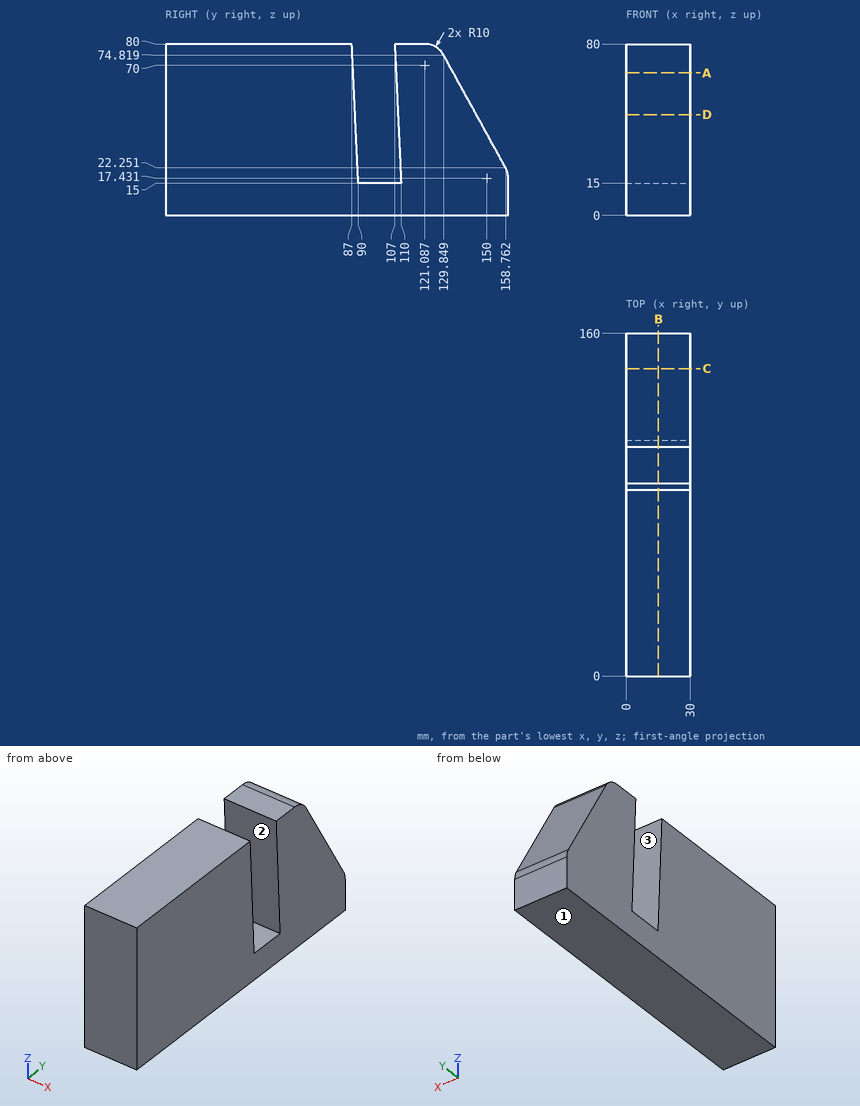
For this review, use the dimensioned drawing (mm, ordinates from the lowest corner) and the shaded views. Give positions to 0.01 mm unless a question says otherwise; leave off trailing zeros. Order: outer loops, then holes, each group sorted by start corner. A loop starts at its lowest first (then second) coordinate and runs counter-clockwise, first axis right, second up. Notation, with made-up numbers: M -29,30 L 28,30 A17 cw 28,35 Z; hole C -32.75,-23 d6. An arc over 180 degrees is marked long. One line per question, with ' | ' between items. Start each with the question number.
1) Mouldability with a two-part tool opening along Z and no side actions: class the marked faces 1, 2 and 3 as pulls with the +Z half, pulls with the -Z half, needs draft (parallel to the pull), parting line crosses it, or undercut.
2) Consider section D-D, the plane z = 47. Give the boundary of the cut face in (x, y), then the cut area to 3 significant figures.
3) Consider section B-B, the plane x = 15. Give the boundary of the cut face in (y, z), then the cut area to 3 significant figures.
4) Clearance check with flat-ended pins moving along their axes: P1, Ø10, axis at x = 10, z = 32.5, coming from the +Y side (1 decimal); P2, Ø5, axis at x = 25, z = 63.5, coming from the +Y side. State where each tip first meets the part, or that it passes through.
5) Consider section A-A, the plane z = 66.5. Give the boundary of the cut face in (x, y) (1 decimal).
6) Wall thickness on L1, parallel to Y at x = 11.25, z = 69; L2, parallel to Y at x = 9.25, z = 46; L3, parallel to Z at x = 18, y = 106.5: over which ranges is each line inside the solid? List them lowest first. Write a range as from..to.
7) Consider section C-C, the plane y = 143.5. Give the boundary of the cut face in (x, z), then the cut area to 3 significant figures.
Found:
1) face 1: pulls with the -Z half | face 2: undercut | face 3: pulls with the +Z half
2) outline: M 0,0 L 30,0 L 30,88.52 L 0,88.52 Z; M 0,108.52 L 30,108.52 L 30,145.15 L 0,145.15 Z | area: 3,750 mm²
3) outline: M 0,0 L 160,0 L 160,17.43 A10 ccw 158.76,22.25 L 129.85,74.82 A10 ccw 121.09,80 L 107,80 L 110,15 L 90,15 L 87,80 L 0,80 Z | area: 10,500 mm²
4) P1: stops at y = 155.9 | P2: stops at y = 137.45
5) outline: M 0,0 L 30,0 L 30,87.6 L 0,87.6 Z; M 0,107.6 L 30,107.6 L 30,134.4 L 0,134.4 Z
6) L1: y = 0..87.51, 107.51..133.05 | L2: y = 0..88.57, 108.57..145.7 | L3: z = 0..15
7) outline: M 0,0 L 30,0 L 30,50 L 0,50 Z | area: 1,500 mm²
